Here's how the part is built. I have some questions about the finished solid (model axes, mm). Face numbers are marked on the shaded views. A direction names the side the tool comes from. Round coordinates to 2 decimals unless told otherwise and drop trailing zeros. Write each loop counter-clockwise with the first axis right and the second up, starting at its lowest first coordinate (ties: lowest second). Pieces come first, ordered by that corner, then holes. Notation, with made-up numbers: (-38, 48) -> (12, 48) arc R17 ccw to (12, 81) -> close; hole circle Ø9 at (69, 79). An arc over 180 degrees is marked (long way). Answer in a Markdown table with one row per item. Add a question column.
from build123d import *
from build123d.topology import SkipClean

# Parameters (mm, degrees)
SKETCH14_R          = 4
SKETCH14_R_2        = 1.2
SKETCH14_R_3        = 5
BOSS_EXTRUDE1_DEPTH = 4
CUT_EXTRUDE1_START  = -2.5
SKETCH15_R          = 1.2
CUT_EXTRUDE1_DEPTH  = 1.5
CUT_EXTRUDE2_DEPTH  = 0.5
SKETCH17_R          = 1
CUT_EXTRUDE3_DEPTH  = 6
SKETCH18_R          = 2.25
CUT_EXTRUDE4_DEPTH  = 10


with BuildPart() as part:
    # Sketch14 → Boss-Extrude1 (new body)
    with BuildSketch(Plane.XY):
        with BuildLine():
            Line((50.08, 3.99919992), (0.1, 4.9989999))
            ThreePointArc((0.1, 4.9989999), (3.570714214, 3.5), (5, 0))
            ThreePointArc((5, 0), (3.570714214, -3.5), (0.1, -4.9989999))
            Line((0.1, -4.9989999), (50.08, -3.99919992))
            ThreePointArc((50.08, -3.99919992), (46, 0), (50.08, 3.99919992))
        make_face()
        with Locations((50, 0)):
            Circle(SKETCH14_R)
        with Locations((50, 0)):
            Circle(SKETCH14_R_2, mode=Mode.SUBTRACT)
        Circle(SKETCH14_R_3)
        Circle(SKETCH14_R_2, mode=Mode.SUBTRACT)
    extrude(amount=BOSS_EXTRUDE1_DEPTH)

    # Sketch15 → Cut-Extrude1 (cut)
    with BuildSketch(Plane.XY.offset(4).offset(CUT_EXTRUDE1_START)):
        with BuildLine():
            Line((16.121698113, 2.33951917), (0.363207547, 3.832829278))
            ThreePointArc((0.363207547, 3.832829278), (-3.85, 0), (0.363207547, -3.832829278))
            Line((0.363207547, -3.832829278), (16.121698113, -2.33951917))
            ThreePointArc((16.121698113, -2.33951917), (18.25, 0), (16.121698113, 2.33951917))
        make_face()
        Circle(SKETCH15_R, mode=Mode.SUBTRACT)
    extrude(amount=-CUT_EXTRUDE1_DEPTH, mode=Mode.SUBTRACT)

    # Sketch16 → Cut-Extrude2 (cut)
    with SkipClean():  # the faces are left unmerged after this step: merging them gives an invalid solid
        with BuildSketch(Plane(origin=(0, 0, 1.5), x_dir=(-1, 0, 0), z_dir=(0, 0, -1))):
            with BuildLine():
                ThreePointArc((-0.363207547, -3.832829278), (-3.85, 0), (-0.363207547, 3.832829278))
                Line((-0.363207547, 3.832829278), (-6, 3.298674112))
                Line((-6, 3.298674112), (-6, -3.298674112))
                Line((-6, -3.298674112), (-0.363207547, -3.832829278))
            make_face()
            with BuildLine():
                ThreePointArc((3.85, 0), (2.722361108, 2.722361108), (0, 3.85))
                Line((0, 3.85), (0, 1.2))
                ThreePointArc((0, 1.2), (0.848528137, 0.848528137), (1.2, 0))
                ThreePointArc((1.2, 0), (0.848528137, -0.848528137), (0, -1.2))
                Line((0, -1.2), (0, -3.85))
                ThreePointArc((0, -3.85), (2.722361108, -2.722361108), (3.85, 0))
            make_face()
            with BuildLine():
                Line((0, 1.2), (0, 3.85))
                ThreePointArc((0, 3.85), (-0.181806598, 3.845704924), (-0.363207547, 3.832829278))
                ThreePointArc((-0.363207547, 3.832829278), (-3.85, 0), (-0.363207547, -3.832829278))
                ThreePointArc((-0.363207547, -3.832829278), (-0.181806598, -3.845704924), (0, -3.85))
                Line((0, -3.85), (0, -1.2))
                ThreePointArc((0, -1.2), (-1.2, 0), (0, 1.2))
            make_face()
        extrude(amount=-CUT_EXTRUDE2_DEPTH, mode=Mode.SUBTRACT)

    # Sketch17 → Cut-Extrude3 (cut)
    with SkipClean():  # the faces are left unmerged after this step: merging them gives an invalid solid
        with BuildSketch(Plane(origin=(0, 0, 1.5), x_dir=(-1, 0, 0), z_dir=(0, 0, -1))):
            with Locations((-11.1, 0)):
                Circle(SKETCH17_R)
        extrude(amount=-CUT_EXTRUDE3_DEPTH, mode=Mode.SUBTRACT)

    # Sketch18 → Cut-Extrude4 (cut)
    with SkipClean():  # the faces are left unmerged after this step: merging them gives an invalid solid
        with BuildSketch(Plane.XY.offset(4)):
            Circle(SKETCH18_R)
        extrude(amount=-CUT_EXTRUDE4_DEPTH, mode=Mode.SUBTRACT)


solid = part.part
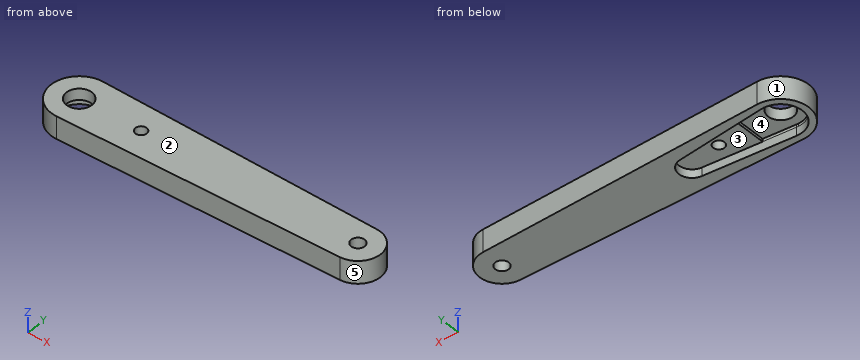
Item 1: On a 3-axis mill with a long thin cutter (end or side, diameter ignored), from which of +Z, -Z, +X, -X, +Y, -Y can I reach the whole of each face in a straight line? I mean the marked faces 4 and 5. Say none if no direction works.
Item 2: If we section it at A-A on z = 2.65: Please give me the cut outline in (x, y).
Item 3: If we section it at C-C on y = 1.75: Please give me the cut outline in (x, z), then the cut area to 3 significant figures.
Item 4: If we section it at D-D on x = -1: Please give me the cut outline in (y, z), then the cut area to 3 significant figures.
Item 5: I need wall thicknesses on line 1 along X through (y, z) = (0.5, 3.6); line 2 along Y through (x, z) = (0, 0.8); line 3 along Y through (x, z) = (11.1, 2.1). Which ranges of each line are inside material? Lowest first, please. Write a range as from..to.
Item 6: For P1, Ø2, axis at x = 9.5, y = -3, coming from the -Z side; P2, Ø2.5, axis at x = 2, y = 0.5, coming from the -Z side; P3, Ø2, axis at x = 14.5, y = 0.5, coming from the -Z side; P4, Ø2.5, axis at x = 0, y = 0, coming from the +Z side, each with a flat end and sliding along its axis, tell me the tip position at first contact or that it passes through.
Item 7: If we section it at B-B on x = 11.1: Please give me the cut outline in (y, z).
Item 8: If we mould it in two halves opening along Y, with no side actions, what happens to the marked faces 1, 2 and 3? For each: pulls with the +Y half, pulls with the -Y half, needs draft (parallel to the pull), parting line crosses it, or undercut.
Results list:
| question | item | result |
|---|---|---|
| 1 | face 4 | -Z |
| 1 | face 5 | +Z, -Z, +X |
| 2 | outline | (0.1, -5) -> (50.08, -4) arc R4 ccw to (50.08, 4) -> (0.1, 5) arc R5 ccw (long way) to start; hole circle Ø4.5 at (0, 0); hole circle Ø2 at (11.1, 0); hole circle Ø2.4 at (50, 0) |
| 3 | outline | (-4.68, 0) -> (-3.43, 0) -> (-3.43, 2) -> (-1.41, 2) -> (-1.41, 4) -> (-4.68, 4) -> close; (1.41, 2) -> (6, 2) -> (6, 1.5) -> (17.47, 1.5) -> (17.47, 0) -> (53.6, 0) -> (53.6, 4) -> (1.41, 4) -> close |
| 3 | area | 191 mm² |
| 4 | outline | (-4.9, 0) -> (-3.72, 0) -> (-3.72, 2) -> (-2.02, 2) -> (-2.02, 4) -> (-4.9, 4) -> close; (2.02, 2) -> (3.72, 2) -> (3.72, 0) -> (4.9, 0) -> (4.9, 4) -> (2.02, 4) -> close |
| 4 | area | 16.3 mm² |
| 5 | line 1 | -4.97..-2.19, 2.19..10.23, 11.97..48.91, 51.09..53.97 |
| 5 | line 2 | -5..-3.85, 3.85..5 |
| 5 | line 3 | -4.78..-1, 1..4.78 |
| 6 | P1 | z = 0 |
| 6 | P2 | z = 2 |
| 6 | P3 | z = 1.5 |
| 6 | P4 | through |
| 7 | outline | (-4.78, 0) -> (-2.82, 0) -> (-2.82, 1.5) -> (-1, 1.5) -> (-1, 4) -> (-4.78, 4) -> close; (1, 1.5) -> (2.82, 1.5) -> (2.82, 0) -> (4.78, 0) -> (4.78, 4) -> (1, 4) -> close |
| 8 | face 1 | parting line crosses it |
| 8 | face 2 | needs draft |
| 8 | face 3 | undercut |
